Read the model definition and answer for the solid it produces. Units are mm, in the model's axes. A direction names the side the tool comes from. Round coordinates to 2 decimals unless told otherwise and drop trailing zeros. Order: outer loops, then holes, each group sorted by start corner. A loop starts at its lowest first (then second) coordinate and runs counter-clockwise, first axis right, second up. Notation, with made-up numbers: (-30, 48.25) - (-19, 48.25) arc R37 ccw to (-19, 84.25) - close; hole circle Ø7 at (-15.75, 4.25). An arc over 180 degrees is marked (long way). One line per question, with ' | ' between items. Start each with the question number.
1) For faces 1 (the flat face through (0, 0, -17)), 2 (the flat face through (-2, 57, 22.15)), 3 (the flat face through (-2, -57, 22.15)), 4 (the flat face through (-2, -71.5, 3)), 5 (the flat face through (-5, -1, 8)), determine the directions among +Z, -Z, +X, -X, +Y, -Y from which every point of the face is accessible in a straight line to the end or side of a thin tool.
2) The part is cut by section C-C, the plane x = -3.2. Count the separate pieces of the cut face and the enclosed holes in it, plus the area to 3 significant figures.
3) The mould has two halves that part along Y. Classify faces 6 (the flat face through (-2, 58, -22.15)), 7 (the flat face through (-2.465, -36.286, 29.45)), 8 (the flat face through (-2, 1, -15.25)): pulls with the +Y half, pulls with the -Y half, needs draft (parallel to the pull), parting line crosses it, or undercut.
4) The part is cut by section B-B, the plane y = -63. Give the vertices of the cut face in (x, z), plus the area to 3 significant figures.
5) Flat-ended cylindrical pins translate along their axes: pin 1 (2.5 mm diameter, centred on x = -3.5, y = 57.5, fed in from +Z); pin 2 (1.5 mm diameter, centred on x = -2, y = 0.5, fed in from -Z). Find the tip coordinate at first contact, or state that the pin passes through.
6) Straight lines are drawn through the part: line 1 (Y direction, x = -2, z = -18.25); line 2 (Z direction, x = -1.95, y = 0); line 3 (Z direction, x = -0.95, y = -65.5). For each, find the intervals that lie inside material, in ascending order. Write a range as from..to.
7) The part is cut by section A-A, the plane z = -4. Give the vertices of the cut face in (x, y).
Autodesk Inventor part; units mm, degrees
ref_plane "YZ Plane" through (0, 0, 0) normal (1, 0, 0) x (0, 1, 0)
ref_plane "XZ Plane" through (0, 0, 0) normal (0, 1, 0) x (-1, 0, 0)
ref_plane "XY Plane" through (0, 0, 0) normal (0, 0, 1) x (1, 0, 0)
sketch "Sketch1" plane through (0, 0, 0) normal (1, 0, 0) x (0, 1, 0)
  line L0 (-73.5, -22.15) -> (73.5, -22.15) construction
  line L1 (73.5, 22.15) -> (-73.5, 22.15) construction
  line L2 (-73.5, 22.15) -> (-73.5, -22.15) construction
  line L3 (-73.5, -22.15) -> (73.5, 22.15) construction
  line L4 (73.5, -22.15) -> (-73.5, 22.15) construction
  line L5 (-73.5, 0) -> (73.5, 0) construction
  line L6 (0, 22.15) -> (0, -22.15) construction
  line L7 (49.5, -18.25) -> (65.5, -18.25) construction
  line L8 (45, -22.15) -> (45, -14.25) construction
  line L9 (45, -14.25) -> (70, -14.25) construction
  line L10 (70, -14.25) -> (70, -22.15) construction
  line L11 (57.5, -14.25) -> (57.5, -22.15) construction
  line L12 (-49.5, -18.25) -> (-65.5, -18.25) construction
  line L13 (-45, -22.15) -> (-45, -14.25) construction
  line L14 (-45, -14.25) -> (-70, -14.25) construction
  line L15 (-70, -14.25) -> (-70, -22.15) construction
  line L16 (-57.5, -14.25) -> (-57.5, -22.15) construction
  line L17 (-73.5, 17.15) -> (69, 17.15) construction
  line L18 (45, -22.15) -> (45, -19.85)
  line L19 (45, -19.85) -> (-45, -19.85)
  line L20 (-45, -19.85) -> (-45, -22.15)
  line L21 (-70, -20.35) -> (70, -20.35) construction
  line L22 (73.5, 22.15) -> (73.5, -22.15) construction
  line L23 (70, -22.15) -> (70, -19.85)
  line L24 (70, -19.85) -> (73.5, -19.85)
  line L25 (-70, -22.15) -> (-70, -19.85)
  line L26 (-70, -19.85) -> (-73.5, -19.85)
  line L27 (71.5, 20.15) -> (71.5, 8.9)
  line L28 (71.5, -15.25) -> (-71.5, -15.25)
  line L29 (71.5, 20.15) -> (-71.5, 20.15) construction
  circle A0 centre (49.5, -18.25) radius 3 construction
  line L30 (71.5, 20.15) -> (71.5, -15.25)
  line L31 (-71.5, 20.15) -> (-71.5, -15.25)
  line L32 (73.5, 22.15) -> (73.5, -19.85)
  line L33 (-73.5, 22.15) -> (-73.5, -19.85)
  line L34 (70, -22.15) -> (45, -22.15)
  line L35 (-45, -22.15) -> (-70, -22.15)
  arc A1 (72.1213, -19.85) -> (70, -21.9713) centre (71.0607, -20.9107) ccw
  arc A2 (45, -21.9713) -> (42.8787, -19.85) centre (43.9393, -20.9107) ccw
  arc A3 (-70, -21.9713) -> (-72.1213, -19.85) centre (-71.0607, -20.9107) ccw
  arc A4 (-42.8787, -19.85) -> (-45, -21.9713) centre (-43.9393, -20.9107) ccw
  line L36 (73.5, 23.15) -> (-73.5, 23.15) construction
  line L37 (43.5858, 22.15) -> (28.5858, 37.15)
  line L38 (28.5858, 37.15) -> (-28.5858, 37.15)
  line L39 (-28.5858, 37.15) -> (-43.5858, 22.15)
  line L40 (-44, 23.15) -> (-29, 38.15) construction
  line L41 (-29, 38.15) -> (29, 38.15) construction
  line L42 (29, 38.15) -> (44, 23.15) construction
  line L43 (42.7574, 20.15) -> (27.7574, 35.15)
  line L44 (27.7574, 35.15) -> (3.7417, 35.15)
  arc A5 (-3.7417, 35.15) -> (3.7417, 35.15) centre (0, 32.65) ccw
  line L45 (-42.7574, 20.15) -> (-27.7574, 35.15)
  line L46 (-27.7574, 35.15) -> (-3.7417, 35.15)
  line L47 (-71.5, 20.15) -> (-42.7574, 20.15)
  line L48 (-43.5858, 22.15) -> (-73.5, 22.15)
  line L49 (42.7574, 20.15) -> (71.5, 20.15)
  line L50 (73.5, 22.15) -> (43.5858, 22.15)
  point P0 (0, 0)
  point P1 (-73.5, -22.15)
  point P2 (-45, -22.15)
  point P3 (-45, -22.15)
  point P4 (-73.5, -19.85)
  point P5 (-70, -22.15)
  point P6 (-72.1213, -19.85)
  point P7 (-70, -21.9713)
  point P8 (-45, -21.9713)
  point P9 (-42.8787, -19.85)
  point P10 (42.8787, -19.85)
  point P11 (45, -21.9713)
  point P12 (-45, -19.85)
  point P13 (45, -19.85)
  point P14 (-70, -19.85)
  point P15 (-63.7555, -20)
  point P16 (-39.2445, -20)
  point P17 (39.2445, -20)
  point P18 (63.7555, -20)
  point P19 (71.5, 8.9)
  dimension "d0" = 147
  dimension "d2" = 16
  dimension "d3" = 3.9
  dimension "d4" = 25
  dimension "d5" = 7.9
  dimension "d18" = 5
  dimension "d35" = 2.1
  dimension "d36" = 0.5
  dimension "d38" = 115
  dimension "d47" = 2
  dimension "d50" = 6
  dimension "d53" = 2
  dimension "d56" = 1.5
  dimension "d57" = 42.5
  dimension "d59" = 1
  dimension "d60" = 14
  dimension "d63" = 45
  dimension "d64" = 15
  dimension "d65" = 1
  dimension "d66" = 1
  dimension "d67" = 88
  dimension "d68" = 43.5
  dimension "d69" = 4.5
  dimension "d70" = 2
  dimension "d71" = 2
extrude "Extrusion1" add sketch "Sketch1" against normal blind 5 contours L18 A2 L19 A4 L20 L35 L25 A3 L26 L33 L48 L39 L38 L37 L50 L32 L24 A1 L23 L34 | L27 L30 L28 L31 L47 L45 L46 A5 L44 L43 L49
extrude "Extrusion2" cut sketch "Sketch1" against normal blind 4 contours L27 L30 L28 L31 L47 L45 L46 A5 L44 L43 L49
hole "M3" at (0, 49.5, -18.25) at (0, 65.5, -18.25) at (0, -65.5, -18.25) at (0, -49.5, -18.25) at (0, 0, 32.65) direction (-1, 0, 0) diameter 2.459 end through all
fillet "R2" radius 2 10 edges at (-2, 71.5, -15.25) (-2, -71.5, -15.25) (-2, -71.5, 20.15) (-2.5, -43.5858, 22.15) (-2.5, 43.5858, 22.15) (-2, -27.7574, 35.15) (-2, -3.7417, 35.15) (-2, 3.7417, 35.15) (-2, 27.7574, 35.15) (-2, 71.5, 20.15)
fillet "R4" radius 4 6 edges at (-2.5, 73.5, 22.15) (-2.5, -28.5858, 37.15) (-2.5, 28.5858, 37.15) (-2.5, -73.5, 22.15) (-2, -42.7574, 20.15) (-2, 42.7574, 20.15)
properties part number "TorsoPelvisCoverFrame" material "Acetal Resin, Black"
Values:
1) face 1: +Z, -Z, +X, +Y, -Y | face 2: +Z, +X, -X, +Y | face 3: +Z, +X, -X, -Y | face 4: +X | face 5: +Z, -Z, -X, +Y, -Y
2) separate pieces: 1 | enclosed holes: 6 | area: 1,270 mm^2
3) face 6: needs draft | face 7: pulls with the -Y half | face 8: undercut
4) outline: (-5, -22.15) - (0, -22.15) - (0, -15.25) - (-4, -15.25) - (-4, 20.15) - (0, 20.15) - (0, 22.15) - (-5, 22.15) - close | area: 79.9 mm^2
5) pin 1: stops at z = 22.15 | pin 2: stops at z = -19.85
6) line 1: y = -73.5..-66.73, -64.27..-50.73, -48.27..48.27, 50.73..64.27, 66.73..73.5 | line 2: z = -19.85..-15.25, 28.15..31.42, 33.88..37.15 | line 3: z = -22.15..-19.48, -17.02..-15.25, 20.15..22.15
7) outline: (-5, -73.5) - (0, -73.5) - (0, -71.5) - (-4, -71.5) - (-4, 71.5) - (0, 71.5) - (0, 73.5) - (-5, 73.5) - close
